from build123d import *

# Parameters (mm, degrees)
F0_W     = 4.6228
F0_H     = 4.6228
F0_H_2   = 3.175
F1_DEPTH = 3.175


with BuildPart() as f1:
    # F0 (on Top) → F1 (new body)
    with BuildSketch(Plane.XY):
        Polygon((44.45, -19.05), (44.45, 19.05), (40.4114, 19.05), (35.7886, 19.05), (27.7114, 19.05), (23.0886, 19.05), (15.0114, 19.05), (10.3886, 19.05), (2.3114, 19.05), (-2.3114, 19.05), (-10.3886, 19.05), (-15.0114, 19.05), (-23.0886, 19.05), (-27.7114, 19.05), (-35.7886, 19.05), (-38.1, 19.05), (-40.4114, 19.05), (-44.45, 19.05), (-44.45, -12.7), (-44.45, -19.05), (-40.4114, -19.05), (-38.1, -19.05), (-35.7886, -19.05), (-27.7114, -19.05), (-23.0886, -19.05), (-15.0114, -19.05), (-10.3886, -19.05), (-2.3114, -19.05), (2.3114, -19.05), (10.3886, -19.05), (15.0114, -19.05), (23.0886, -19.05), (27.7114, -19.05), (35.7886, -19.05), (40.4114, -19.05), align=None)
        with Locations((-38.1, -12.7)):
            Rectangle(F0_W, F0_H, mode=Mode.SUBTRACT)
        with Locations((-25.4, -12.7)):
            Rectangle(F0_W, F0_H, mode=Mode.SUBTRACT)
        with Locations((-12.7, -12.7)):
            Rectangle(F0_W, F0_H, mode=Mode.SUBTRACT)
        with Locations((0, -12.7)):
            Rectangle(F0_W, F0_H, mode=Mode.SUBTRACT)
        with Locations((12.7, -12.7)):
            Rectangle(F0_W, F0_H, mode=Mode.SUBTRACT)
        with Locations((25.4, -12.7)):
            Rectangle(F0_W, F0_H, mode=Mode.SUBTRACT)
        with Locations((38.1, -12.7)):
            Rectangle(F0_W, F0_H, mode=Mode.SUBTRACT)
        with Locations((-38.1, 0)):
            Rectangle(F0_W, F0_H, mode=Mode.SUBTRACT)
        with Locations((-25.4, 0)):
            Rectangle(F0_W, F0_H, mode=Mode.SUBTRACT)
        with Locations((-12.7, 0)):
            Rectangle(F0_W, F0_H, mode=Mode.SUBTRACT)
        with Locations((-38.1, 12.7)):
            Rectangle(F0_W, F0_H, mode=Mode.SUBTRACT)
        with Locations((-25.4, 12.7)):
            Rectangle(F0_W, F0_H, mode=Mode.SUBTRACT)
        with Locations((-12.7, 12.7)):
            Rectangle(F0_W, F0_H, mode=Mode.SUBTRACT)
        Rectangle(F0_W, F0_H, mode=Mode.SUBTRACT)
        with Locations((12.7, 0)):
            Rectangle(F0_W, F0_H, mode=Mode.SUBTRACT)
        with Locations((25.4, 0)):
            Rectangle(F0_W, F0_H, mode=Mode.SUBTRACT)
        with Locations((38.1, 0)):
            Rectangle(F0_W, F0_H, mode=Mode.SUBTRACT)
        with Locations((0, 12.7)):
            Rectangle(F0_W, F0_H, mode=Mode.SUBTRACT)
        with Locations((12.7, 12.7)):
            Rectangle(F0_W, F0_H, mode=Mode.SUBTRACT)
        with Locations((25.4, 12.7)):
            Rectangle(F0_W, F0_H, mode=Mode.SUBTRACT)
        with Locations((38.1, 12.7)):
            Rectangle(F0_W, F0_H, mode=Mode.SUBTRACT)
        with Locations((38.1, 20.6375)):
            Rectangle(F0_W, F0_H_2)
        with Locations((38.1, -20.6375)):
            Rectangle(F0_W, F0_H_2)
        with Locations((25.4, 20.6375)):
            Rectangle(F0_W, F0_H_2)
        with Locations((25.4, -20.6375)):
            Rectangle(F0_W, F0_H_2)
        with Locations((12.7, 20.6375)):
            Rectangle(F0_W, F0_H_2)
        with Locations((12.7, -20.6375)):
            Rectangle(F0_W, F0_H_2)
        with Locations((0, 20.6375)):
            Rectangle(F0_W, F0_H_2)
        with Locations((0, -20.6375)):
            Rectangle(F0_W, F0_H_2)
        with Locations((-12.7, 20.6375)):
            Rectangle(F0_W, F0_H_2)
        with Locations((-12.7, -20.6375)):
            Rectangle(F0_W, F0_H_2)
        with Locations((-25.4, 20.6375)):
            Rectangle(F0_W, F0_H_2)
        with Locations((-25.4, -20.6375)):
            Rectangle(F0_W, F0_H_2)
        Polygon((-38.1, 19.05), (-35.7886, 19.05), (-35.7886, 22.225), (-40.4114, 22.225), (-40.4114, 19.05), align=None)
        Polygon((-35.7886, -22.225), (-35.7886, -19.05), (-38.1, -19.05), (-40.4114, -19.05), (-40.4114, -22.225), align=None)
    extrude(amount=F1_DEPTH)


solid = f1.part
Design review of the part built by this model. Coordinates are the model's own, in mm. A direction names the side the tool comes from. Round coordinates to 2 decimals unless told otherwise and drop trailing zeros. Write each loop counter-clockwise with the first axis right and the second up, starting at its lowest first coordinate (ties: lowest second). Pieces come first, ordered by that corner, then holes. Notation, with made-up numbers: (32.5, 33.5) -> (58.5, 33.5) arc R22 cw to (58.5, 41.5) -> close; hole circle Ø3 at (-22, 79.25). An arc over 180 degrees is marked (long way). One line per item, written item: value. Start each with the question number.
Q1. The part is to be moulded in two halves that separate along Y. For faces 1 (the face through (0, -22.225, 2)), 2 (the face through (42, 19.05, 2)), 3 (the face through (-35.789, 21, 2)), 4 (the face through (10.389, -13, 2)), say which applies: pulls with the +Y half, pulls with the -Y half, needs draft (parallel to the pull), parting line crosses it, or undercut.
Q2. Insertion check: P1, Ø1.6, axis at y = 20.5, z = 1.5, coming from the +X side; P2, Ø1, axis at x = 19, z = 1.5, coming from the +Y side. Each pin has a flat end and moves straight along its axis. Give the tip position at first contact, or say it passes through.
Q3. Tool access review of faces 5 (the face through (13, -22.225, 2)), 6 (the face through (-23.089, -21, 2)), 7 (the face through (-23.089, 0, 2)), 8 (the face through (-42, 19.05, 2)), 9 (the face through (-27.711, 21, 2)): name each direction out of +Z, -Z, +X, -X, +Y, -Y from which nothing blocks a thin tool from reaching the whole face with its end or side.
Q4. Add section A-A (y = -12.5). State how many separate pieces and enclosed holes the cut face has, then the cut area to 3 significant figures.
Q5. To check wall thickness, follow probe 1 along Y at (x, z) = (-0.5, 2.45) (3 decimals); probe 2 along Y at (x, z) = (-9, 0.25). State the ranges of each line that lie inside material, in increasing order.
Q6. Add section C-C (x = 34). Give the boundary of the cut face in (y, z) (3 decimals), then the cut area to 3 significant figures.
Response:
1. face 1: pulls with the -Y half
1. face 2: pulls with the +Y half
1. face 3: needs draft
1. face 4: undercut
2. P1: stops at x = 40.41
2. P2: stops at y = 19.05
3. face 5: +Z, -Z, +X, -X, -Y
3. face 6: +Z, -Z, -Y
3. face 7: +Z, -Z
3. face 8: +Z, -Z, -X, +Y
3. face 9: +Z, -Z, +Y
4. separate pieces: 8
4. enclosed holes: 0
4. area: 180 mm^2
5. probe 1: y = -22.225 to -15.011, -10.389 to -2.311, 2.311 to 10.389, 15.011 to 22.225
5. probe 2: y = -19.05 to 19.05
6. outline: (-19.05, 0) -> (19.05, 0) -> (19.05, 3.175) -> (-19.05, 3.175) -> close
6. area: 121 mm^2
